Autodesk Inventor part; units mm, degrees
ref_plane "YZ Plane" through (0, 0, 0) normal (1, 0, 0) x (0, 1, 0)
ref_plane "XZ Plane" through (0, 0, 0) normal (0, 1, 0) x (-1, 0, 0)
ref_plane "XY Plane" through (0, 0, 0) normal (0, 0, 1) x (1, 0, 0)
sketch "スケッチ1" plane through (0, 0, 0) normal (0, 0, 1) x (1, 0, 0)
  circle A0 centre (0, 0) radius 3
  dimension "d0" = 6
extrude "押し出し1" add sketch "スケッチ1" along normal blind 55
hole "穴1" at (0, 0, 0) direction (0, 0, 1) diameter 3 depth 6 tip angle 118
sketch "スケッチ2" plane through (0, 0, 55) normal (0, 0, 1) x (1, 0, 0)
  circle A0 centre (0, 0) radius 3
hole "穴2" at (0, 0, 55) direction (0, 0, -1) diameter 3 depth 6 tip angle 118
properties part number "スペーサ　m3-l55" material "アルミニウム 2014-T4"
Build history of the part. All positions in model axes, mm. A direction names the side the tool comes from. Give positions to 0.01 mm unless a question says otherwise; leave off trailing zeros. Order: outer loops, then holes, each group sorted by start corner. A loop starts at its lowest first (then second) coordinate and runs counter-clockwise, first axis right, second up. Notation, with made-up numbers: M -17.75,-33 L 35.25,-33 A32 cw 35.25,6 Z; hole C -1.5,-19 d9. An arc over 180 degrees is marked long. Write item = value, one per line. Start each with the question number.
(1) Slice it at C-C on x = 2.05. Write the cut outline in (y, z).
(2) Slice it at A-A on z = 5. Write the cut outline in (x, y), plus the area to 3 significant figures.
(3) Probe L1, parallel to Y at x = 0, z = 1.85; L2, parallel to X at y = -0.2, z = 33; L3, parallel to Y at x = 0.5, z = 27.5. List the from-to ranges inside material, lowest first. Write a range as [from, to].
(4) Two-plate mould, pull along X, no slides. Class faces 3 (the flat face through (1.3, -1.3, 55)), 4 (the conical face through (0.078, -0.248, 48.255)), 5 (the cylindrical face through (-0.07, 1.5, 51.96)), 6 (the cylindrical face through (-3, 0, 27)): released by +X, released by -X, zero draft, split by the parting line, or undercut.
(5) Pin check, flat tips, straight feed: pin 1 Ø1.5 at (y, z) = (1, 22.5) entering from +X; pin 2 Ø2.5 at (x, y) = (0, 0) entering from +Z; pin 3 Ø1 at (x, z) = (1, 41) entering from -Y. Stop position of each tip, or through.
(6) Which spindle directions (+Z, -Z, +X, -X, +Y, -Y) get a long thin tool onto all of the face, cutting with end or side? Do faces 1 (the cylindrical face through (-0.07, -1.5, 3.04)), 2 (the flat face through (1.3, -1.3, 0)). Say none if no direction does.
(7) Slice it at B-B on z = 27.5. Write the cut outline in (x, y).
Responses:
q1.outline = M -2.19,0 L 2.19,0 L 2.19,55 L -2.19,55 Z
q2.outline = C 0,0 d6; hole C 0,0 d3
q2.area = 21.2 mm2
q3.L1 = [-3, -1.5], [1.5, 3]
q3.L2 = [-2.99, 2.99]
q3.L3 = [-2.96, 2.96]
q4.face_3 = zero draft
q4.face_4 = undercut
q4.face_5 = undercut
q4.face_6 = split by the parting line
q5.pin_1 = 2.99
q5.pin_2 = 48.85
q5.pin_3 = -2.96
q6.face_1 = -Z
q6.face_2 = -Z, +X, -X, +Y, -Y
q7.outline = C 0,0 d6
